The listing builds one solid part. Answer for the finished solid, in the listing's coordinates (mm). A direction names the side the tool comes from. Give positions to 0.01 mm unless a question says otherwise; leave off trailing zeros. Write each loop counter-clockwise with the first axis right and the second up, starting at its lowest first coordinate (ties: lowest second). Pieces come first, ordered by that corner, then holes. Notation, with made-up numbers: (-37.5, 25.5) -> (-27.5, 25.5) arc R8 cw to (-27.5, 33.5) -> close; hole circle Ø3 at (-12.5, 18). An arc over 180 degrees is marked (long way). One line per question, with ' | ' between items.
from build123d import *

# Parameters (mm, degrees)
SKETCH1_R                 = 4.7371
SKETCH1_R_2               = 2.5
BOSS_EXTRUDE1_DEPTH       = 6.35
SKETCH2_R                 = 3.175
SKETCH2_R_2               = 2.5
BOSS_EXTRUDE2_DEPTH       = 33.02
F_4_40_TAPPED_HOLE1_D     = 2.2606
F_4_40_TAPPED_HOLE1_DEPTH = 4.7361
F_4_40_TAPPED_HOLE1_TIP   = 0.679152758


with BuildPart() as part:
    # Sketch1 → Boss-Extrude1 (new body)
    with BuildSketch(Plane.XY):
        Circle(SKETCH1_R)
        Circle(SKETCH1_R_2, mode=Mode.SUBTRACT)
    extrude(amount=BOSS_EXTRUDE1_DEPTH)

    # Sketch2 → Boss-Extrude2 (add)
    with BuildSketch(Plane.XY.offset(6.35)):
        Circle(SKETCH2_R)
        Circle(SKETCH2_R_2, mode=Mode.SUBTRACT)
    extrude(amount=BOSS_EXTRUDE2_DEPTH)

    # #4-40 Tapped Hole1
    with Locations(Plane.ZY.offset(4.7371)):
        with Locations((3.191608174, 0)):
            Hole(F_4_40_TAPPED_HOLE1_D / 2, depth=F_4_40_TAPPED_HOLE1_DEPTH)
            with Locations((0, 0, -(F_4_40_TAPPED_HOLE1_DEPTH + F_4_40_TAPPED_HOLE1_TIP / 2))):  # 118° drill point
                Cone(0, F_4_40_TAPPED_HOLE1_D / 2, F_4_40_TAPPED_HOLE1_TIP, mode=Mode.SUBTRACT)


solid = part.part
Item 1: Consider line 1 (Y direction, x = -0.5, z = 24); line 2 (X direction, y = 1.75, z = 19). Determine where each line is inside the solid, lowest interval first. Write a range as [from, to].
Answers below:
line 1: [-3.14, -2.45], [2.45, 3.14] | line 2: [-2.65, -1.79], [1.79, 2.65]
Item 2: Find section C-C (z = 20). Write down the section's boundary in (x, y) (3 decimals).
Answers below:
outline: circle Ø6.35 at (0, 0); hole circle Ø5 at (0, 0)
Item 3: Find section B-B (y = 0). Write down the section's boundary in (x, z) (3 decimals).
Answers below:
outline: (-4.737, 0) -> (-2.5, 0) -> (-2.5, 2.061) -> (-4.737, 2.061) -> close; (-4.737, 4.322) -> (-2.5, 4.322) -> (-2.5, 39.37) -> (-3.175, 39.37) -> (-3.175, 6.35) -> (-4.737, 6.35) -> close; (2.5, 0) -> (4.737, 0) -> (4.737, 6.35) -> (3.175, 6.35) -> (3.175, 39.37) -> (2.5, 39.37) -> close
Item 4: Determine the mould class of faces 4 (the face through (-0.54, -2.44, 19.41)), 5 (the face through (0, -3, 39.37)), 6 (the face through (4.376, -1.814, 3.131)) for opening direction X: pulls with the +X half, pulls with the -X half, needs draft (parallel to the pull), parting line crosses it, or undercut.
Answers below:
face 4: undercut | face 5: needs draft | face 6: parting line crosses it
Item 5: A tool of negligible diameter and unlimited length cuts with its end or side. For faces 1 (the face through (-3.466, -0.433, 2.147)), 2 (the face through (2, -2, 0)), 3 (the face through (-0.69, -3.1, 22.63)), from which of +Z, -Z, +X, -X, +Y, -Y can it reach the whole face along a straight path? Write none if from no direction.
Answers below:
face 1: -X | face 2: -Z, +X, -X, +Y, -Y | face 3: +Z
Item 6: Flat-ended cylindrical pins translate along their axes: pin 1 (5 mm diameter, centred on x = 1, z = 17, fed in from -Y) (3 decimals); pin 2 (1 mm diameter, centred on y = 1, z = 19, fed in from +X); pin 3 (1.5 mm diameter, centred on y = 0.5, z = 23.5, fed in from -X) (3 decimals). Find the tip coordinate at first contact, or state that the pin passes through.
Answers below:
pin 1: y = -3.175 | pin 2: x = 3.14 | pin 3: x = -3.175
Item 7: Find section A-A (x = 0). Write down the section's boundary in (y, z) (3 decimals), then the cut area to 3 significant figures.
Answers below:
outline: (-4.737, 0) -> (-2.5, 0) -> (-2.5, 39.37) -> (-3.175, 39.37) -> (-3.175, 6.35) -> (-4.737, 6.35) -> close; (2.5, 0) -> (4.737, 0) -> (4.737, 6.35) -> (3.175, 6.35) -> (3.175, 39.37) -> (2.5, 39.37) -> close | area: 73.0 mm²
Item 8: Find section D-D (x = 1.5). Write down the section's boundary in (y, z).
Answers below:
outline: (-4.49, 0) -> (-2, 0) -> (-2, 39.37) -> (-2.8, 39.37) -> (-2.8, 6.35) -> (-4.49, 6.35) -> close; (2, 0) -> (4.49, 0) -> (4.49, 6.35) -> (2.8, 6.35) -> (2.8, 39.37) -> (2, 39.37) -> close
